```python
from build123d import *

# Parameters (mm, degrees)
SKETCH1_W           = 148
SKETCH1_H           = 214
BOSS_EXTRUDE1_DEPTH = 89
SKETCH2_W           = 5.566237362
SKETCH2_H           = 3.86389192
CUT_EXTRUDE1_DEPTH  = 212
SKETCH3_W           = 24.825910207
SKETCH3_H           = 52.918387546
BOSS_EXTRUDE2_DEPTH = 5
FILLET1_R           = 1
SKETCH4_W           = 125
SKETCH4_H           = 29
BOSS_EXTRUDE3_DEPTH = 1
LPATTERN1_COUNT     = 3
LPATTERN1_PITCH     = 29.5


with BuildPart() as part:
    # Sketch1 → Boss-Extrude1 (new body)
    with BuildSketch(Plane(origin=(0, 0, 0), x_dir=(1, 0, 0), z_dir=(0, 1, 0))):
        Rectangle(SKETCH1_W, SKETCH1_H)
    extrude(amount=BOSS_EXTRUDE1_DEPTH)

    # Sketch2 → Cut-Extrude1 (cut)
    with BuildSketch(Plane.XY.offset(107)):
        with Locations((-74, 44.5)):
            Rectangle(SKETCH2_W, SKETCH2_H)
    cut_extrude1 = extrude(amount=-CUT_EXTRUDE1_DEPTH, mode=Mode.SUBTRACT)

    # Mirror1: Cut-Extrude1 across plane
    add(cut_extrude1.mirror(Plane(origin=(0, 0, 0), x_dir=(0, 0, 1), z_dir=(1, 0, 0))), mode=Mode.SUBTRACT)

    # Sketch3 → Boss-Extrude2 (add)
    with BuildSketch(Plane.XY.offset(107)):
        with Locations((-53.45043607, 49.977386193)):
            Rectangle(SKETCH3_W, SKETCH3_H)
    extrude(amount=BOSS_EXTRUDE2_DEPTH)

    # Fillet1
    fillet1_edges = [part.edges().sort_by_distance(p)[0] for p in [
        (-41.037480966, 49.977386193, 107),
        (-41.037480966, 23.51819242, 109.5),
        (-53.450436069, 76.436579966, 107),
        (-41.037480966, 76.436579966, 109.5),
        (-65.863391173, 49.977386193, 107),
        (-65.863391173, 76.436579966, 109.5),
        (-53.450436069, 23.51819242, 107),
        (-65.863391173, 23.51819242, 109.5),
        (-41.037480966, 49.977386193, 112),
        (-53.450436069, 76.436579966, 112),
        (-65.863391173, 49.977386193, 112),
        (-53.450436069, 23.51819242, 112),
    ]]
    fillet(fillet1_edges, radius=FILLET1_R)

    # Sketch4 → Boss-Extrude3 (add)
    with BuildSketch(Plane(origin=(0, 0, -107), x_dir=(-1, 0, 0), z_dir=(0, 0, -1))):
        with Locations((-4.420464609, 74)):
            Rectangle(SKETCH4_W, SKETCH4_H)
    boss_extrude3 = extrude(amount=BOSS_EXTRUDE3_DEPTH)

    # LPattern1: Boss-Extrude3 ×3
    with Locations(*[(0, -i * LPATTERN1_PITCH, 0) for i in range(1, LPATTERN1_COUNT)]):
        add(boss_extrude3)


solid = part.part
```
Input: part model. Units: mm. Frame: model coordinates. Coordinates: 2 decimals unless noted, no trailing zeros. Order: outer loops, then holes, each group sorted by start corner. A loop starts at its lowest first (then second) coordinate and runs counter-clockwise, first axis right, second up. Notation, with made-up numbers: (75, -3) - (81, -3) arc R15 cw to (81, 10) - close; hole circle Ø8 at (60, 45). An arc over 180 degrees is marked (long way). Put each result on its own line as item: value.
1. Line query: line 1 along Z through (x, y) = (12.5, 54); line 2 along X through (y, z) = (46, -23.5); line 3 along Z through (x, y) = (-66, 27). Output: solid intervals per line, ascending.
Report:
line 1: z = -108 to 107
line 2: x = -71.22 to 71.22
line 3: z = -107 to 107.5
2. Contact query for flat-ended pins moving along their axis: pin 1 Ø3 at (x, y) = (73, 45.5) entering from +Z; pin 2 Ø2 at (x, y) = (-46, 22) entering from +Z; pin 3 Ø0.5 at (x, z) = (21, -107.5) entering from -Y. Output: stop coordinate, or through.
Report:
pin 1: stops at z = 107
pin 2: stops at z = 107.12
pin 3: stops at y = 0.5
3. Cut plane A-A on y = 7. Return the cut outline in (x, z).
Report:
outline: (-74, -107) - (-58.08, -107) - (-58.08, -108) - (66.92, -108) - (66.92, -107) - (74, -107) - (74, 107) - (-74, 107) - close
4. Cut plane C-C on y = 70. Return the cut outline in (x, z), then the cut area to 3 significant figures.
Report:
outline: (-74, -107) - (-58.08, -107) - (-58.08, -108) - (66.92, -108) - (66.92, -107) - (74, -107) - (74, 107) - (-40.04, 107) arc R1 cw to (-41.04, 108) - (-41.04, 111) arc R1 ccw to (-42.04, 112) - (-64.86, 112) arc R1 ccw to (-65.86, 111) - (-65.86, 108) arc R1 cw to (-66.86, 107) - (-74, 107) - close
area: 31,900 mm2
5. Cut plane B-B on x = 47. Return the cut outline in (y, z).
Report:
outline: (0, -107) - (0.5, -107) - (0.5, -108) - (29.5, -108) - (29.5, -107) - (30, -107) - (30, -108) - (59, -108) - (59, -107) - (59.5, -107) - (59.5, -108) - (88.5, -108) - (88.5, -107) - (89, -107) - (89, 107) - (0, 107) - close
